from build123d import *


with BuildPart() as part:
    # Sketch1 → Revolve1 (revolve)
    with BuildSketch(Plane.XY):
        with BuildLine():
            Line((-6.3, 26), (4.726601718, 14.973398282))
            ThreePointArc((4.726601718, 14.973398282), (11.450917759, 11.091112606), (19.215489112, 11.091112606))
            Line((19.215489112, 11.091112606), (65.619388603, 23.525))
            Line((65.619388603, 23.525), (65.619388603, 26))
            Line((65.619388603, 26), (8, 26))
            Line((8, 26), (8, 32))
            Line((8, 32), (0, 32))
            Line((0, 32), (0, 26))
            Line((0, 26), (-6.3, 26))
        make_face()
    revolve(axis=Axis((0, 0, 0), (1, 0, 0)))


solid = part.part
Here's how the part is built. I have some questions about the finished solid (model axes, mm). A direction names the side the tool comes from. Coordinates: 2 decimals unless noted, no trailing zeros. Write each loop counter-clockwise with the first axis right and the second up, starting at its lowest first coordinate (ties: lowest second). Pieces come first, ordered by that corner, then holes.
Item 1: I want a section at D-D on z = 27.5. Write out the boundary of the cut face in (x, y), and give its area (3 significant figures).
Item 2: I want a section at A-A on y = 0. Write out the boundary of the cut face in (x, z) (3 decimals), and give its area (3 significant figures).
Item 3: If I drill on line 1 (X direction, y = 28, z = -15); line 2 (Y direction, x = 41.5, z = -8); line 3 (Y direction, x = 43.5, z = -1), over which ranges is the centre line in solid material (lowest first)?
Item 4: If we mould it in two halves opening along Y, with no side actions, what happens to faces 1 (the flat face through (65.619, 6, -23)), 2 (the cylindrical face through (-3.194, -20.633, -15.821)), 3 (the conical face through (37.586, 15.274, 4.81))? For each: +Y half, -Y half, draft (parallel to the pull), parting line (faces both ways), or undercut.
Item 5: Will these pins go through, and if not, where does the flat tip stop? pin 1 (5 mm diameter, centred on y = -23.5, z = -22.5, fed in from +X); pin 2 (1.5 mm diameter, centred on y = -12, z = 0, fed in from -X); pin 3 (3 mm diameter, centred on x = 18.5, y = -13.5, fed in from -Z).
Item 6: I want a section at C-C on x = 54.5. Write out the boundary of the cut face in (y, z).
Item 7: On a 3-axis mill with a long thin cutter (end or side, diameter ignored), from which of +Z, -Z, +X, -X, +Y, -Y can I reach the whole of each face in a straight line? I mean faces 4 (the cylindrical face through (3.94, -6.94, -31.24)), 5 (the flat face through (0, -0.1, 26.2)), 6 (the flat face through (8, 0.1, 26.2)). Say none if no direction works.
Findings below:
1. outline: (0, -16.36) - (8, -16.36) - (8, 16.36) - (0, 16.36) - close
1. area: 262 mm2
2. outline: (-6.3, -26) - (0, -26) - (0, -32) - (8, -32) - (8, -26) - (65.619, -26) - (65.619, -23.525) - (19.215, -11.091) arc R15 ccw to (4.727, -14.973) - close; (-6.3, 26) - (4.727, 14.973) arc R15 ccw to (19.215, 11.091) - (65.619, 23.525) - (65.619, 26) - (8, 26) - (8, 32) - (0, 32) - (0, 26) - close
2. area: 1,440 mm2
3. line 1: x = 0 to 8
3. line 2: y = -24.74 to -15.07, 15.07 to 24.74
3. line 3: y = -25.98 to -17.57, 17.57 to 25.98
4. face 1: draft
4. face 2: parting line
4. face 3: undercut
5. pin 1: stops at x = 8
5. pin 2: stops at x = 7.56
5. pin 3: stops at z = -23.07
6. outline: circle Ø52 at (0, 0); hole circle Ø41.09 at (0, 0)
7. face 4: +X, -X
7. face 5: -X
7. face 6: +X
